from build123d import *

# Parameters (mm, degrees)
SKETCH1_W           = 20
SKETCH1_H           = 23
BOSS_EXTRUDE1_DEPTH = 2
SKETCH2_W           = 10.5
SKETCH2_H           = 4
SKETCH2_W_2         = 5.5
SKETCH2_H_2         = 3
SKETCH2_R           = 1.5
CUT_EXTRUDE1_DEPTH  = 10


with BuildPart() as part:
    # Sketch1 → Boss-Extrude1 (new body)
    with BuildSketch(Plane.XY):
        Rectangle(SKETCH1_W, SKETCH1_H)
    extrude(amount=BOSS_EXTRUDE1_DEPTH)

    # Sketch2 → Cut-Extrude1 (cut)
    with BuildSketch(Plane.XY.offset(2)):
        with Locations((0, 2.5)):
            Rectangle(SKETCH2_W, SKETCH2_H)
        with Locations((-2.5, -7.5)):
            Rectangle(SKETCH2_W_2, SKETCH2_H_2)
        with Locations((2.25, -6)):
            Circle(SKETCH2_R)
    extrude(amount=-CUT_EXTRUDE1_DEPTH, mode=Mode.SUBTRACT)


solid = part.part
Geometry check sheet. Reference: the model listing, model coordinates, mm. A direction names the side the tool comes from. Give positions to 0.01 mm unless a question says otherwise; leave off trailing zeros. Order: outer loops, then holes, each group sorted by start corner. A loop starts at its lowest first (then second) coordinate and runs counter-clockwise, first axis right, second up.
1. Sectioned sample at A-A (x = -1.25). Record the boundary of the cut face in (y, z), then the cut area to 3 significant figures.
Completed:
outline: (-11.5, 0) - (-9, 0) - (-9, 2) - (-11.5, 2) - close; (-6, 0) - (0.5, 0) - (0.5, 2) - (-6, 2) - close; (4.5, 0) - (11.5, 0) - (11.5, 2) - (4.5, 2) - close
area: 32.0 mm2
2. Draft check along X on faces 1 (the face through (0, 0, 2)), 2 (the face through (-10, 0, 1)), 3 (the face through (0.25, -8, 1)), 4 (the face through (-3, -9, 1)). Enter one of: pulls with the +X half, pulls with the -X half, needs draft (parallel to the pull), parting line crosses it, or undercut.
Completed:
face 1: needs draft
face 2: pulls with the -X half
face 3: undercut
face 4: undercut
3. Sectioned sample at C-C (z = 0.65). Record the boundary of the cut face in (x, y), then the cut area to 3 significant figures.
Completed:
outline: (-10, -11.5) - (10, -11.5) - (10, 11.5) - (-10, 11.5) - close; hole (-5.25, -9) - (0.25, -9) - (0.25, -6) - (-5.25, -6) - close; hole (-5.25, 0.5) - (5.25, 0.5) - (5.25, 4.5) - (-5.25, 4.5) - close; hole circle Ø3 at (2.25, -6)
area: 394 mm2
4. Depth check by flat-ended pin: pin 1 (8 mm diameter, centred on x = 2, y = -6.5, fed in from -Z). Enter the tip coordinate at first touch or a pass-through.
Completed:
pin 1: stops at z = 0
5. Access from +Z, -Z, +X, -X, +Y, -Y to the whole of each face (thin tool, end or side, straight path). Record for faces 5 (the face through (10, 0, 1)), 6 (the face through (5.25, 2, 1)).
Completed:
face 5: +Z, -Z, +X, +Y, -Y
face 6: +Z, -Z
6. Scan lines: line 1 (Y direction, x = 2.25, z = 1); line 2 (Y direction, x = -4.5, z = 1.85); line 3 (X direction, y = 3, z = 1.45). Record each from-to range of solid material in increasing order.
Completed:
line 1: y = -11.5 to -7.5, -4.5 to 0.5, 4.5 to 11.5
line 2: y = -11.5 to -9, -6 to 0.5, 4.5 to 11.5
line 3: x = -10 to -5.25, 5.25 to 10
7. Sectioned sample at B-B (y = 4). Record the boundary of the cut face in (x, z).
Completed:
outline: (-10, 0) - (-5.25, 0) - (-5.25, 2) - (-10, 2) - close; (5.25, 0) - (10, 0) - (10, 2) - (5.25, 2) - close
8. Sectioned sample at D-D (x = 3). Record the boundary of the cut face in (y, z).
Completed:
outline: (-11.5, 0) - (-7.3, 0) - (-7.3, 2) - (-11.5, 2) - close; (-4.7, 0) - (0.5, 0) - (0.5, 2) - (-4.7, 2) - close; (4.5, 0) - (11.5, 0) - (11.5, 2) - (4.5, 2) - close
